Autodesk Inventor part; units mm, degrees
ref_plane "body_to_dummy_XY" through (0, 0, 0) normal (0, -1, 0) x (1, 0, 0)
ref_plane "body_to_dummy_YZ" through (0, 0, 0) normal (1, 0, 0) x (0, 0, 1)
ref_plane "body_to_dummy_ZX" through (0, 0, 0) normal (0, 0, 1) x (0, -1, 0)
sketch "Sketch_1" plane through (0, 0, 0) normal (0, 1, 0) x (1, 0, 0)
  line L0 (-2.54, 1.27) -> (-2.54, -1.27)
  line L1 (-2.54, -1.27) -> (2.54, -1.27)
  line L2 (2.54, -1.27) -> (2.54, 1.27)
  line L3 (2.54, 1.27) -> (-2.54, 1.27)
extrude "Extrusion1" add sketch "Sketch_1" along normal blind 6.096
sketch "Sketch_2" plane through (0, 5.461, 0) normal (0, 1, 0) x (1, 0, 0)
  line L0 (-2.794, 2.54) -> (-2.794, -2.54)
  line L1 (-2.794, -2.54) -> (2.794, -2.54)
  line L2 (2.794, -2.54) -> (2.794, 2.54)
  line L3 (2.794, 2.54) -> (-2.794, 2.54)
  line L4 (-2.286, 1.016) -> (-2.286, -1.016)
  line L5 (-2.286, -1.016) -> (2.286, -1.016)
  line L6 (2.286, -1.016) -> (2.286, 1.016)
  line L7 (2.286, 1.016) -> (-2.286, 1.016)
extrude "Extrusion2" cut sketch "Sketch_2" against normal blind 0.508
sketch "Sketch_3" plane through (0, 6.096, 0) normal (0, 1, 0) x (1, 0, 0)
  line L0 (-0.762, 1.27) -> (-0.762, -1.27)
  line L1 (-0.762, -1.27) -> (0.762, -1.27)
  line L2 (0.762, -1.27) -> (0.762, 1.27)
  line L3 (0.762, 1.27) -> (-0.762, 1.27)
extrude "Extrusion3" cut sketch "Sketch_3" against normal blind 2.54
sketch "Sketch_4" plane through (0, 6.096, 0) normal (0, 1, 0) x (1, 0, 0)
  line L0 (-1.778, 0.4445) -> (-1.778, -0.4445)
  line L1 (-1.778, -0.4445) -> (1.778, -0.4445)
  line L2 (1.778, -0.4445) -> (1.778, 0.4445)
  line L3 (1.778, 0.4445) -> (-1.778, 0.4445)
extrude "Extrusion4" cut sketch "Sketch_4" against normal blind 6.096
sketch "Sketch_5" plane through (0, 5.7912, 0) normal (0, 1, 0) x (1, 0, 0)
  line L0 (-2.032, 0.5969) -> (-2.032, -0.5969)
  line L1 (-2.032, -0.5969) -> (2.032, -0.5969)
  line L2 (2.032, -0.5969) -> (2.032, 0.5969)
  line L3 (2.032, 0.5969) -> (-2.032, 0.5969)
extrude "Extrusion5" cut sketch "Sketch_5" against normal blind 6.096
sketch "Sketch_8" plane through (0, 0, 0) normal (0, 1, 0) x (-1, 0, 0)
  line L0 (0.762, -0.6477) -> (0.762, 0.6477)
  line L1 (0.762, 0.6477) -> (-0.762, 0.6477)
  line L2 (-0.762, 0.6477) -> (-0.762, -0.6477)
  line L3 (-0.762, -0.6477) -> (0.762, -0.6477)
extrude "Extrusion6" cut sketch "Sketch_8" along normal blind 3.556
sketch "Sketch_6" plane through (0, 0, 0) normal (1, 0, 0) x (0, 1, 0)
  line L0 (3.0093, 0.2159) -> (2.2752, -0.6477)
  line L1 (2.2752, -0.6477) -> (6.096, -0.6477)
  line L2 (6.096, -0.6477) -> (6.096, 0.2159)
  line L3 (6.096, 0.2159) -> (3.0093, 0.2159)
extrude "Extrusion7" add sketch "Sketch_6" along normal mid plane 1.27
sketch "Sketch_7" plane through (0, 0, 0) normal (1, 0, 0) x (0, 1, 0)
  line L0 (6.096, 1.27) -> (6.096, -1.27)
  line L1 (6.096, -1.27) -> (8.636, -0.635)
  line L2 (8.636, -0.635) -> (11.557, -0.635)
  line L3 (11.557, -0.635) -> (11.557, -0.508)
  line L4 (11.557, -0.508) -> (11.811, -0.508)
  line L5 (11.811, -0.508) -> (11.811, -0.635)
  line L6 (11.811, -0.635) -> (12.319, -0.635)
  line L7 (12.319, -0.635) -> (12.319, -0.508)
  line L8 (12.319, -0.508) -> (12.573, -0.508)
  line L9 (12.573, -0.508) -> (12.573, -0.635)
  line L10 (12.573, -0.635) -> (13.081, -0.635)
  line L11 (13.081, -0.635) -> (13.081, -0.508)
  line L12 (13.081, -0.508) -> (13.335, -0.508)
  line L13 (13.335, -0.508) -> (13.335, -0.635)
  line L14 (13.335, -0.635) -> (13.97, -0.635)
  line L15 (13.97, -0.635) -> (13.97, 0.635)
  line L16 (13.97, 0.635) -> (13.335, 0.635)
  line L17 (13.335, 0.635) -> (13.335, 0.508)
  line L18 (13.335, 0.508) -> (13.081, 0.508)
  line L19 (13.081, 0.508) -> (13.081, 0.635)
  line L20 (13.081, 0.635) -> (12.573, 0.635)
  line L21 (12.573, 0.635) -> (12.573, 0.508)
  line L22 (12.573, 0.508) -> (12.319, 0.508)
  line L23 (12.319, 0.508) -> (12.319, 0.635)
  line L24 (12.319, 0.635) -> (11.811, 0.635)
  line L25 (11.811, 0.635) -> (11.811, 0.508)
  line L26 (11.811, 0.508) -> (11.557, 0.508)
  line L27 (11.557, 0.508) -> (11.557, 0.635)
  line L28 (11.557, 0.635) -> (8.636, 0.635)
  line L29 (8.636, 0.635) -> (6.096, 1.27)
extrude "Extrusion8" add sketch "Sketch_7" along normal mid plane 5.08
sketch "Sketch_10" plane through (0, 0, 0) normal (1, 0, 0) x (0, 1, 0)
  line L0 (8.636, 1.27) -> (6.096, 1.27)
  line L1 (6.096, 1.27) -> (6.096, -1.27)
  line L2 (6.096, -1.27) -> (8.636, -1.27)
  line L3 (8.636, -1.27) -> (8.636, 1.27)
extrude "Extrusion9" cut sketch "Sketch_10" along normal mid plane 3.81
ref_plane "body_to_dummy_XY" through (0, 0, 0) normal (0, -1, 0) x (1, 0, 0)
ref_plane "body_to_dummy_YZ" through (0, 0, 0) normal (1, 0, 0) x (0, 0, 1)
ref_plane "body_to_dummy_ZX" through (0, 0, 0) normal (0, 0, 1) x (0, -1, 0)
properties part number "SNT-100-BK-H_body"
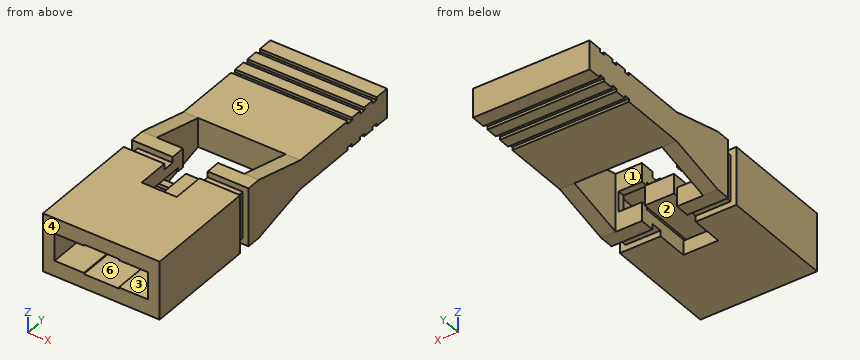
Here's how the part is built. I have some questions about the finished solid (model axes, mm). Face numbers are marked on the shaded views. A direction names the side the tool comes from. Give positions to 0.01 mm unless a question says otherwise; leave off trailing zeros. Write each loop counter-clockwise with the first axis right and the second up, starting at its lowest first coordinate (ties: lowest second). Pieces come first, ordered by that corner, then holes. Notation, with made-up numbers: (82, 73.25) -> (138, 73.25) arc R16 cw to (138, 85.25) -> close; hole circle Ø1 at (-18.5, 48.25). An arc over 180 degrees is marked (long way). Use one line per item in the form item = value. Start each with the question number.
1. If I drill on L1, parallel to X at y = 5.5, z = -0.55 (3 decimals); L2, parallel to Z at x = -1.2, y = 4.25; L3, parallel to X at y = 7.5, z = 0.7 (3 decimals), over which ranges is the centre line in solid material (lowest first)?
2. Thinking about a two-plate mould opening in Z: for the marked faces 4, 5 and 6, which applies, +Z half, -Z half, draft (parallel to the pull), parting line (faces both ways), or undercut?
3. Imagine slicing it at D-D on z = -0.8. List the corners of the cut face in (x, y) for me (3 decimals).
4. Imagine slicing it at C-C on x = -0.1. State how many separate pieces and enclosed holes the cut face has, plus the area to 3 significant figures.
5. On a 3-axis mill with a long thin cutter (end or side, diameter ignored), from which of +Z, -Z, +X, -X, +Y, -Y can I reach the whole of each face in a straight line? I mean the marked faces 1, 2 and 3. Say none if no direction works.
6. Will this pin go through, and if not, where does the flat tip stop? pin 1 Ø1 at (x, z) = (-1.5, 0) entering from -Y.
7. Imagine slicing it at B-B on z = 0.05. List the corners of the cut face in (x, y) for me (3 decimals).
8. Imagine slicing it at A-A on y = 7.5. List the corners of the cut face in (x, z) for me (3 decimals).
Entries:
q1.L1 = -2.54 to -2.032, -0.635 to 0.635, 2.032 to 2.54
q1.L2 = -1.27 to -0.6, 0.6 to 1.27
q1.L3 = -2.54 to -1.905, 1.905 to 2.54
q2.face_4 = draft
q2.face_5 = +Z half
q2.face_6 = undercut
q3.outline = (-2.54, 0) -> (2.54, 0) -> (2.54, 4.953) -> (2.286, 4.953) -> (2.286, 5.461) -> (2.54, 5.461) -> (2.54, 7.976) -> (1.905, 7.976) -> (1.905, 6.096) -> (0.762, 6.096) -> (0.762, 3.556) -> (-0.762, 3.556) -> (-0.762, 6.096) -> (-1.905, 6.096) -> (-1.905, 7.976) -> (-2.54, 7.976) -> (-2.54, 5.461) -> (-2.286, 5.461) -> (-2.286, 4.953) -> (-2.54, 4.953) -> close
q4.separate_pieces = 3
q4.enclosed_holes = 0
q4.area = 14.0 mm²
q5.face_1 = +Z, -Z
q5.face_2 = -Z, +Y
q5.face_3 = -Y
q6.pin_1 = 5.79
q7.outline = (-2.54, 0) -> (-2.032, 0) -> (-2.032, 5.791) -> (-1.778, 5.791) -> (-1.778, 6.096) -> (-1.905, 6.096) -> (-1.905, 8.636) -> (1.905, 8.636) -> (1.905, 6.096) -> (1.778, 6.096) -> (1.778, 5.791) -> (2.032, 5.791) -> (2.032, 0) -> (2.54, 0) -> (2.54, 4.953) -> (2.286, 4.953) -> (2.286, 5.461) -> (2.54, 5.461) -> (2.54, 13.97) -> (-2.54, 13.97) -> (-2.54, 5.461) -> (-2.286, 5.461) -> (-2.286, 4.953) -> (-2.54, 4.953) -> close; (-0.635, 2.868) -> (0.635, 2.868) -> (0.635, 6.096) -> (-0.635, 6.096) -> close
q8.outline = (-2.54, -0.919) -> (-1.905, -0.919) -> (-1.905, 0.919) -> (-2.54, 0.919) -> close; (1.905, -0.919) -> (2.54, -0.919) -> (2.54, 0.919) -> (1.905, 0.919) -> close
